Work out the finished part from the listing and answer in its coordinate system (mm). Face numbers are marked on the shaded views. Give positions to 0.01 mm unless a question says otherwise; leave off trailing zeros. Loops run counter-clockwise (first coordinate to the right, second up) from the corner with the lowest first, then second, coordinate; pieces in that order, holes last. Notation, with made-up numbers: M -25,80.5 L 17,80.5 A15 ccw 17,90.5 Z; hole C -27,5.5 d4. An arc over 180 degrees is marked long. Write item = value, one per line. Start each with the question number.
1. Consider L1, parallel to X at y = 46, z = 0; L2, parallel to Y at x = 41, z = -7; L3, parallel to X at y = 62, z = -1. Determine where each line is inside the solid, lowest interval first. Write a range as [from, to].
2. Section A-A on x = 0 is taken. Determine the outline of the cut face in (y, z).
3. Section C-C on y = 44 is taken. Determine the outline of the cut face in (x, z).
4. Section B-B on z = 0 is taken. Determine the outline of the cut face in (x, y), plus the area to 3 significant figures.
5. Section D-D on x = 44.5 is taken. Determine the outline of the cut face in (y, z), plus the area to 3 significant figures.
6. The mould has two halves that part along Z. Classify the marked faces 1, 2 and 3: released by +Z, released by -Z, zero draft, split by the parting line, or undercut.
7. Flat-ended cylindrical pins translate along their axes: pin 1 Ø4 at (x, y) = (-26.5, 23) entering from -Z; pin 2 Ø12 at (x, y) = (-20.5, 67) entering from +Z; pin 3 Ø1 at (y, z) = (64, -5.5) entering from +X. Find the tip coordinate at first contact, or state that the pin passes through.
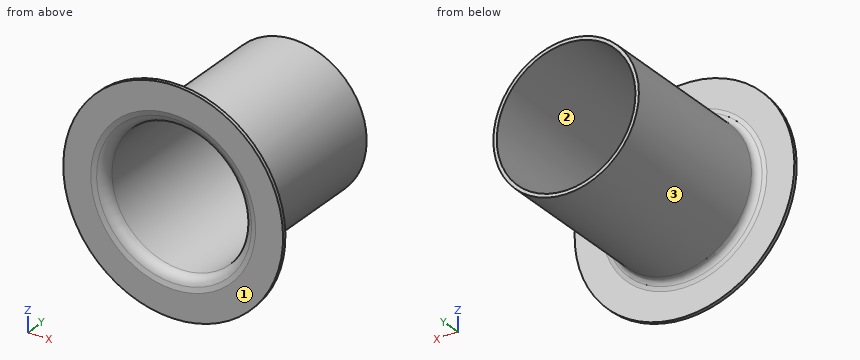
```python
from build123d import *


with BuildPart() as part:
    # Sketch2 → Revolve1 (revolve)
    with BuildSketch(Plane.XY, mode=Mode.PRIVATE) as revolve1_sk:
        with BuildLine():
            Line((38.1, 0), (50.8, 0))
            Line((50.8, 0), (50.8, 1.5875))
            Line((50.8, 1.5875), (38.1, 1.5875))
            Line((38.1, 1.5875), (36.216874251, 2.092082024))
            ThreePointArc((36.216874251, 2.092082024), (34.360110092, 3.332732171), (33.6423, 5.447332512))
            Line((33.6423, 5.447332512), (33.6423, 81.647332512))
            Line((33.6423, 81.647332512), (32.0548, 81.647332512))
            Line((32.0548, 81.647332512), (32.0548, 5.517827557))
            ThreePointArc((32.0548, 5.517827557), (33.104565031, 2.425319498), (35.819999251, 0.610924359))
            Line((35.819999251, 0.610924359), (38.1, 0))
        make_face()
    revolve(revolve1_sk.sketch.rotate(Axis((0, 0, 0), (0, 1, 0)), 90), axis=Axis((0, 0, 0), (0, 1, 0)))


solid = part.part
```
Verdict:
q1.L1 = [-33.64, -32.05], [32.05, 33.64]
q1.L2 = [0, 1.59]
q1.L3 = [-33.63, -32.04], [32.04, 33.63]
q2.outline = M 0,-50.8 L 1.59,-50.8 L 1.59,-38.1 L 2.09,-36.22 A3.47 cw 5.45,-33.64 L 81.65,-33.64 L 81.65,-32.05 L 5.52,-32.05 A5.08 ccw 0.61,-35.82 L 0,-38.1 Z; M 0,38.1 L 0.61,35.82 A5.08 ccw 5.52,32.05 L 81.65,32.05 L 81.65,33.64 L 5.45,33.64 A3.47 cw 2.09,36.22 L 1.59,38.1 L 1.59,50.8 L 0,50.8 Z
q3.outline = C 0,0 d67.28; hole C 0,0 d64.11
q4.outline = M -50.8,0 L -38.1,0 L -35.82,0.61 A5.08 ccw -32.05,5.52 L -32.05,81.65 L -33.64,81.65 L -33.64,5.45 A3.47 cw -36.22,2.09 L -38.1,1.59 L -50.8,1.59 Z; M 32.05,5.52 A5.08 ccw 35.82,0.61 L 38.1,0 L 50.8,0 L 50.8,1.59 L 38.1,1.59 L 36.22,2.09 A3.47 cw 33.64,5.45 L 33.64,81.65 L 32.05,81.65 Z
q4.area = 306 mm2
q5.outline = M 0,-24.5 L 1.59,-24.5 L 1.59,24.5 L 0,24.5 Z
q5.area = 77.8 mm2
q6.face_1 = zero draft
q6.face_2 = undercut
q6.face_3 = split by the parting line
q7.pin_1 = -23.06
q7.pin_2 = 30.36
q7.pin_3 = 33.27
